from build123d import *

# Parameters (mm, degrees)
SKETCH_W             = 50
SKETCH_H             = 6.2
PAD_DEPTH            = 4
SKETCH001_W          = 50
SKETCH001_H          = 2.25
POCKET_DEPTH         = 2
PAD001_DEPTH         = 2.25
SKETCH003_W          = 58.610697
SKETCH003_H          = 2.473083
POCKET001_DEPTH      = 5
POCKET001_DEPTH_BACK = -5


with BuildPart() as part:
    # Sketch → Pad (new body)
    with BuildSketch(Plane.XY):
        with Locations((25, 3.1)):
            Rectangle(SKETCH_W, SKETCH_H)
    extrude(amount=PAD_DEPTH)

    # Sketch001 (on Face6 of Pad) → Pocket (cut)
    with BuildSketch(Plane.XY.offset(4)):
        with Locations((25, 3.125)):
            Rectangle(SKETCH001_W, SKETCH001_H)
    extrude(amount=-POCKET_DEPTH, mode=Mode.SUBTRACT)

    # Sketch002 (on Face8 of Pocket) → Pad001 (join)
    with BuildSketch(Plane.XZ.offset(-4.25)):
        with BuildLine():
            Line((5.8, 2), (10.2, 2))
            Line((10.2, 2), (10.2, 8.9))
            ThreePointArc((5.8, 8.9), (8, 6.7), (10.2, 8.9))
            Line((5.8, 8.9), (5.8, 2))
        make_face()
        with BuildLine():
            Line((13.8, 2), (18.2, 2))
            Line((18.2, 2), (18.2, 8.9))
            ThreePointArc((13.8, 8.9), (16, 6.7), (18.2, 8.9))
            Line((13.8, 8.9), (13.8, 2))
        make_face()
        with BuildLine():
            ThreePointArc((31.8, 8.9), (34, 6.7), (36.2, 8.9))
            Line((36.2, 8.9), (36.2, 2))
            Line((36.2, 2), (31.8, 2))
            Line((31.8, 2), (31.8, 8.9))
        make_face()
        with BuildLine():
            ThreePointArc((39.8, 8.9), (42, 6.7), (44.2, 8.9))
            Line((44.2, 8.9), (44.2, 2))
            Line((44.2, 2), (39.8, 2))
            Line((39.8, 2), (39.8, 8.9))
        make_face()
    extrude(amount=PAD001_DEPTH)

    # Sketch003 (on Face17 of Pad001) → Pocket001 (cut, two sides)
    with BuildSketch(Plane(origin=(0, 2, 0), x_dir=(-1, 0, 0), z_dir=(0, 1, 0))) as pocket001_sk:
        with Locations((-25.710698, 9.085399)):
            Rectangle(SKETCH003_W, SKETCH003_H)
    extrude(amount=-POCKET001_DEPTH, mode=Mode.SUBTRACT)
    extrude(pocket001_sk.sketch, amount=-POCKET001_DEPTH_BACK, mode=Mode.SUBTRACT)


solid = part.part
The model under review builds one solid part; all positions refer to its coordinate system, in mm. A direction names the side the tool comes from. Round coordinates to 2 decimals unless told otherwise and drop trailing zeros. Loops run counter-clockwise (first coordinate to the right, second up) from the corner with the lowest first, then second, coordinate; pieces in that order, holes last. Notation, with made-up numbers: M 70.5,45 L 82.5,45 A28 cw 82.5,71 Z; hole C -13.5,40 d2. An arc over 180 degrees is marked long. Answer as a JSON object with one key per item and string values.
Item 1: For line 1 along X through (y, z) = (3.5, 4); line 2 along Y through (x, z) = (5.5, 2.5); line 3 along Z through (x, y) = (28, 1.5), list the stretches that pass through material, from the lowest coordinate up.
Check sheet entries:
{"line 1": "5.8 to 10.2, 13.8 to 18.2, 31.8 to 36.2, 39.8 to 44.2", "line 2": "0 to 2, 4.25 to 6.2", "line 3": "0 to 4"}
Item 2: Tool access review of faces 1 (the face through (34, 4.25, 6)), 2 (the face through (12, 3, 2)), 3 (the face through (16, 3.1, 6.7)), 4 (the face through (44.2, 3, 5)), 5 (the face through (3, 3, 2)): name each direction out of +Z, -Z, +X, -X, +Y, -Y from which nothing blocks a thin tool from reaching the whole face with its end or side.
Check sheet entries:
{"face 1": "+Z, +X, -X, +Y", "face 2": "+Z", "face 3": "+Z, +Y, -Y", "face 4": "+Z, +X", "face 5": "+Z, -X"}
Item 3: The part is to be moulded in two halves that separate along Y. For faces 6 (the face through (34, 3.1, 6.7)), 7 (the face through (8, 2, 6)), 8 (the face through (16, 4.25, 6)), 9 (the face through (18.2, 3, 5)), say which applies: +Y half, -Y half, draft (parallel to the pull), parting line (faces both ways), or undercut.
Check sheet entries:
{"face 6": "draft", "face 7": "-Y half", "face 8": "+Y half", "face 9": "undercut"}
Item 4: We need section C-C, the plane y = 2.5. State the section outline as (x, z) points.
Check sheet entries:
{"outline": "M 0,0 L 50,0 L 50,2 L 44.2,2 L 44.2,7.85 L 43.93,7.85 A2.2 cw 40.07,7.85 L 39.8,7.85 L 39.8,2 L 36.2,2 L 36.2,7.85 L 35.93,7.85 A2.2 cw 32.07,7.85 L 31.8,7.85 L 31.8,2 L 18.2,2 L 18.2,7.85 L 17.93,7.85 A2.2 cw 14.07,7.85 L 13.8,7.85 L 13.8,2 L 10.2,2 L 10.2,7.85 L 9.93,7.85 A2.2 cw 6.07,7.85 L 5.8,7.85 L 5.8,2 L 0,2 Z"}
Item 5: We need section B-B, the plane z = 5.25. State the section outline as (x, y) points, and give its area (3 significant figures).
Check sheet entries:
{"outline": "M 5.8,2 L 10.2,2 L 10.2,4.25 L 5.8,4.25 Z; M 13.8,2 L 18.2,2 L 18.2,4.25 L 13.8,4.25 Z; M 31.8,2 L 36.2,2 L 36.2,4.25 L 31.8,4.25 Z; M 39.8,2 L 44.2,2 L 44.2,4.25 L 39.8,4.25 Z", "area": "39.6 mm2"}
Item 6: We need section A-A, the plane z = 3. State the section outline as (x, y) points, and give its area (3 significant figures).
Check sheet entries:
{"outline": "M 0,0 L 50,0 L 50,2 L 44.2,2 L 44.2,4.25 L 50,4.25 L 50,6.2 L 0,6.2 L 0,4.25 L 5.8,4.25 L 5.8,2 L 0,2 Z; hole M 10.2,2 L 13.8,2 L 13.8,4.25 L 10.2,4.25 Z; hole M 18.2,2 L 31.8,2 L 31.8,4.25 L 18.2,4.25 Z; hole M 36.2,2 L 39.8,2 L 39.8,4.25 L 36.2,4.25 Z", "area": "237 mm2"}
Item 7: We need section D-D, the plane x = 21. State the section outline as (y, z) points, and give its area (3 significant figures).
Check sheet entries:
{"outline": "M 0,0 L 6.2,0 L 6.2,4 L 4.25,4 L 4.25,2 L 2,2 L 2,4 L 0,4 Z", "area": "20.3 mm2"}
Item 8: Clearance check with flat-ended pins moving along their axes: P1, Ø2.5, axis at x = 48.5, y = 2.5, coming from the +Z side; P2, Ø1.2, axis at x = 16.5, z = 5.5, coming from the -Y side; P3, Ø0.6, axis at x = 38, z = 3, coming from the -Y side; P4, Ø1.8, axis at y = 3, z = 5, coming from the +X side. State where each tip first meets the part, or that it passes through.
Check sheet entries:
{"P1": "z = 4", "P2": "y = 2", "P3": "y = 0", "P4": "x = 44.2"}
